Build history of the part. All positions in model axes, mm. A direction names the side the tool comes from. Round coordinates to 2 decimals unless told otherwise and drop trailing zeros. Write each loop counter-clockwise with the first axis right and the second up, starting at its lowest first coordinate (ties: lowest second). Pieces come first, ordered by that corner, then holes. Notation, with made-up numbers: (58, -14.75) - (71, -14.75) arc R21 ccw to (71, 18.25) - close; hole circle Ø1 at (11, 45). An arc over 180 degrees is marked (long way). One line per question, with ' | ' between items.
from build123d import *

# Parameters (mm, degrees)
SKETCH1_R           = 1.27
BOSS_EXTRUDE1_DEPTH = 2.54
CHAMFER1_SIZE       = 0.762
SKETCH2_W           = 46.799762806
SKETCH2_H           = 2.54
CUT_EXTRUDE1_DEPTH  = 5.334


with BuildPart() as part:
    # Sketch1 → Boss-Extrude1 (new body)
    with BuildSketch(Plane.XY):
        Polygon((-104.877780152, -24.027219848), (-50.8, -24.027219848), (-50.8, 24.027219848), (-104.877780152, 24.027219848), (-107.95, 20.955), (-107.95, -20.955), align=None)
        with Locations((-101.009537176, 21.805359873)):
            Circle(SKETCH1_R, mode=Mode.SUBTRACT)
        with Locations((-79.51282161, 21.805359873)):
            Circle(SKETCH1_R, mode=Mode.SUBTRACT)
        with Locations((-53.676916467, 21.805359873)):
            Circle(SKETCH1_R, mode=Mode.SUBTRACT)
        with Locations((-53.676916467, 0)):
            Circle(SKETCH1_R, mode=Mode.SUBTRACT)
        with Locations((-53.676916467, -21.805359873)):
            Circle(SKETCH1_R, mode=Mode.SUBTRACT)
        with Locations((-79.51282161, -21.805359873)):
            Circle(SKETCH1_R, mode=Mode.SUBTRACT)
        with Locations((-101.009537176, -21.805359873)):
            Circle(SKETCH1_R, mode=Mode.SUBTRACT)
        with Locations((-105.440631813, -8.320112928)):
            Circle(SKETCH1_R, mode=Mode.SUBTRACT)
        with Locations((-105.440631813, 8.320112928)):
            Circle(SKETCH1_R, mode=Mode.SUBTRACT)
    extrude(amount=BOSS_EXTRUDE1_DEPTH)

    # Chamfer1
    chamfer1_edges = [part.edges().sort_by_distance(p)[0] for p in [
        (-80.78282161, 21.805359873, 2.54),
        (-54.946916467, 21.805359873, 2.54),
        (-102.279537176, 21.805359873, 2.54),
        (-54.946916467, 0, 2.54),
        (-54.946916467, -21.805359873, 2.54),
        (-80.78282161, -21.805359873, 2.54),
        (-102.279537176, -21.805359873, 2.54),
        (-106.710631813, -8.320112928, 2.54),
        (-106.710631813, 8.320112928, 2.54),
    ]]
    chamfer(chamfer1_edges, length=CHAMFER1_SIZE)

    # Sketch2 → Cut-Extrude1 (cut)
    with BuildSketch(Plane.XY.offset(2.54)):
        with Locations((-81.583109387, 0)):
            Rectangle(SKETCH2_W, SKETCH2_H)
    extrude(amount=-CUT_EXTRUDE1_DEPTH, mode=Mode.SUBTRACT)


solid = part.part
Q1. Pull direction Y, two halves, no side cores. Call faces 1 (the flat face through (-50.8, 0, 1)), 2 (the flat face through (-78, -24.027, 1)), 3 (the cylindrical face through (-101.9, -20.9, 0.9)): +Y half, -Y half, draft (parallel to the pull), parting line (faces both ways), or undercut.
Found:
face 1: draft | face 2: -Y half | face 3: undercut
Q2. Drill centre lines: L1, parallel to Y at x = -97.5, z = 1.5; L2, parallel to X at y = 0.5, z = 0.6; L3, parallel to X at y = 22.5, z = 1.9 (3 decimals). Where is each one in solid material? Low to high. Write a range as from..to.
Found:
L1: -24.03..-1.27, 1.27..24.03 | L2: -107.95..-104.98, -58.18..-54.84, -52.51..-50.8 | L3: -106.405..-102.216, -99.803..-80.719, -78.307..-54.883, -52.471..-50.8
Q3. Drop flat-ended pins along their axis: pin 1 (4 mm diameter, centred on x = -53.68, y = -21.81, fed in from -Z); pin 2 (3.5 mm diameter, centred on x = -79.51, y = -21.81, fed in from +Z). Give the stop position or say it passes through.
Found:
pin 1: z = 0 | pin 2: z = 2.26
Q4. Saw through at C-C, the plane z = 0.4. State how many separate pieces and enclosed holes the cut face has, then the cut area to 3 significant figures.
Found:
separate pieces: 1 | enclosed holes: 10 | area: 2,570 mm^2
Q5. Which spindle directions (+Z, -Z, +X, -X, +Y, -Y) get a long thin tool onto all of the face, cutting with end or side? Do faces 4 (the flat face through (-80, 6, 2.54)), 5 (the flat face through (-104.983, 0, 1)). Say none if no direction does.
Found:
face 4: +Z, +X, -X, +Y, -Y | face 5: +Z, -Z
Q6. Saw through at B-B, the plane x = -67.5. List the corners of the cut face in (y, z), then the cut area to 3 significant figures.
Found:
outline: (-24.03, 0) - (-1.27, 0) - (-1.27, 2.54) - (-24.03, 2.54) - close; (1.27, 0) - (24.03, 0) - (24.03, 2.54) - (1.27, 2.54) - close | area: 116 mm^2
Q7. Saw through at A-A, the plane y = 0. List the corners of the cut face in (x, z), then the cut area to 3 significant figures.
Found:
outline: (-107.95, 0) - (-104.98, 0) - (-104.98, 2.54) - (-107.95, 2.54) - close; (-58.18, 0) - (-54.95, 0) - (-54.95, 1.78) - (-55.71, 2.54) - (-58.18, 2.54) - close; (-52.41, 0) - (-50.8, 0) - (-50.8, 2.54) - (-51.64, 2.54) - (-52.41, 1.78) - close | area: 19.3 mm^2
